Build history of the part. All positions in model axes, mm. A direction names the side the tool comes from. Coordinates: 2 decimals unless noted, no trailing zeros. Write each loop counter-clockwise with the first axis right and the second up, starting at its lowest first coordinate (ties: lowest second). Pieces come first, ordered by that corner, then holes. Notation, with made-up numbers: (85.5, 15.25) -> (107.5, 15.25) arc R24 ccw to (107.5, 26.25) -> close; hole circle Ø9 at (35.25, 13.25). An arc over 180 degrees is marked (long way). Write each question's results on one line, items separated by ' | '. Start each with the question number.
Q1. Saw through at D-D on x = 28.5. Give the cut face in (y, z) (3 decimals).
Q2. Drop flat-ended pins along their axis: pin 1 Ø1.6 at (x, z) = (20.5, 2) entering from +Y; pin 2 Ø0.8 at (y, z) = (16, 1.5) entering from -X (3 decimals); pin 3 Ø1.3 at (y, z) = (10, 1.5) entering from +X. Give the stop position or say it passes through.
Q3. Drill centre lines: line 1 (Y direction, x = 8.65, z = 1.3) (3 decimals); line 2 (X direction, y = 26.5, z = 1.1) (3 decimals); line 3 (Y direction, x = 10, z = 0.7) (3 decimals). Where is each one in solid material? Low to high.
Q4. Saw through at C-C on z = 2.65. Count the separate pieces of the cut face and the enclosed holes in it, and give its area (3 significant figures).
Q5. Saw through at B-B on x = 18.5. Give the cut face in (y, z) (3 decimals).
Q6. Tool access for faces 1 (the face through (8.5, 16, 2)), 2 (the face through (3.175, 30, 2)), 3 (the face through (6, 15, 2)), 4 (the face through (7, 34, 2)), 5 (the face through (10.8, 28, 2)): list every direction of +Z, -Z, +X, -X, +Y, -Y with a clear straight run to the whole face (end or side of a thin tool).
Q7. Saw through at A-A on y = 22.5. Give the cut face in (x, z) (3 decimals), and give its area (3 significant figures).
Q8. Two-plate mould, pull along X, no slides. Class faces 6 (the face through (0, 3, 2)), 7 (the face through (37, 34, 2)), 8 (the face through (8.5, 10, 2)): released by +X, released by -X, zero draft, split by the parting line, or undercut.
from build123d import *

# Parameters (mm, degrees)
SKETCH1_R           = 1.1
BOSS_EXTRUDE1_DEPTH = 3.175
CHAMFER1_SIZE       = 15


with BuildPart() as part:
    # Sketch1 → Boss-Extrude1 (new body)
    # profile 1 of 6: a face of its own
    with BuildSketch(Plane.XY):
        Polygon((10.8, 21.8), (10.8, 34), (3.175, 34), (3.175, 26.1), (3.175, 26), (0, 26), (0, 19.9), (3.175, 19.9), (3.175, 19.8), (3.175, 17), (40, 17), (40, 34), (34, 34), (34, 21.8), align=None)
        with Locations((8.65, 27.9)):
            Circle(SKETCH1_R, mode=Mode.SUBTRACT)
        with Locations((36.15, 27.9)):
            Circle(SKETCH1_R, mode=Mode.SUBTRACT)
    # profile 2 of 6: a face of its own
    with BuildSketch(Plane.XY):
        Polygon((40, 0), (40, 17), (3.175, 17), (3.175, 15), (8.5, 15), (8.5, 16.625), (12, 16.625), (12, 15), (20, 15), (20, 11), (12, 11), (12, 9.375), (8.5, 9.375), (8.5, 11), (3.175, 11), (3.175, 6.2), (3.175, 6.1), (0, 6.1), (0, 0), align=None)
    # profile 3 of 6: a face of its own
    with BuildSketch(Plane.XY):
        Polygon((3.175, 26), (3.175, 26.1), (0, 26), align=None)
    # profile 4 of 6: a face of its own
    with BuildSketch(Plane.XY):
        Polygon((3.175, 19.9), (0, 19.9), (3.175, 19.8), align=None)
    # profile 5 of 6: a face of its own
    with BuildSketch(Plane.XY):
        Polygon((3.175, 6.2), (0, 6.1), (3.175, 6.1), align=None)
    # profile 6 of 6: a face of its own
    with BuildSketch(Plane.XY):
        Polygon((40, -0.1), (40, 0), (0, 0), (3.175, -0.1), align=None)
    extrude(amount=BOSS_EXTRUDE1_DEPTH)

    # Chamfer1
    chamfer1_edges = [part.edges().sort_by_distance(p)[0] for p in [
        (40, -0.1, 1.5875),
    ]]
    chamfer(chamfer1_edges, length=CHAMFER1_SIZE)


solid = part.part
Returned:
1) outline: (3.4, 0) -> (21.8, 0) -> (21.8, 3.175) -> (3.4, 3.175) -> close
2) pin 1: stops at y = 21.8 | pin 2: stops at x = 3.175 | pin 3: stops at x = 35.75
3) line 1: y = -0.1 to 9.375, 16.625 to 26.8, 29 to 34 | line 2: x = 3.175 to 10.8, 34 to 40 | line 3: y = -0.1 to 9.375, 16.625 to 34
4) separate pieces: 1 | enclosed holes: 2 | area: 813 mm2
5) outline: (-0.1, 0) -> (11, 0) -> (11, 3.175) -> (-0.1, 3.175) -> close; (15, 0) -> (21.8, 0) -> (21.8, 3.175) -> (15, 3.175) -> close
6) face 1: +Z, -Z | face 2: +Z, -Z, -X, +Y | face 3: +Z, -Z, -X | face 4: +Z, -Z, +X, -X, +Y | face 5: +Z, -Z, +Y
7) outline: (0, 0) -> (10.8, 0) -> (10.8, 3.175) -> (0, 3.175) -> close; (34, 0) -> (40, 0) -> (40, 3.175) -> (34, 3.175) -> close | area: 53.3 mm2
8) face 6: released by -X | face 7: zero draft | face 8: undercut
